Part model, mm, in its own coordinate system. Face numbers are marked on the shaded views. A direction names the side the tool comes from. Give positions to 0.01 mm unless a question says otherwise; leave off trailing zeros. Write each loop counter-clockwise with the first axis right and the second up, starting at its lowest first coordinate (ties: lowest second). Pieces come first, ordered by that corner, then holes. Notation, with made-up numbers: (60.5, 75.25) - (107.5, 75.25) arc R32 cw to (107.5, 108.25) - close; hole circle Ø5 at (74.5, 43). An arc over 180 degrees is marked (long way). Answer in a Markdown table with one row per item. Add a question column.
1. Drop flat-ended pins along their axis: pin 1 Ø4.5 at (x, y) = (0, 0) entering from +Z; pin 2 Ø5 at (x, y) = (0, 0) entering from -Z; pin 3 Ø3 at (y, z) = (12.5, -0.5) entering from -X. Give the stop position or say it passes through.
2. Band-saw the part on A-A on z = -2. Write the cut outline in (x, y).
3. Probe line 1 along Y through (x, z) = (0, 4.05); line 2 along Y through (x, z) = (0, 5.6); line 3 along X through (y, z) = (0, 3.25). List the from-to ranges inside material, lowest first.
4. Which spindle directions (+Z, -Z, +X, -X, +Y, -Y) get a long thin tool onto all of the face, cutting with end or side? Do the marked faces 1 and 2. Say none if no direction does.
5. Band-saw the part on C-C on x = -14.5. Write the cut outline in (y, z).
6. Pull direction Y, two halves, no side cores. Call the marked faces 3, 4 and 5: released by +Y, released by -Y, zero draft, split by the parting line, or undercut.
7. Band-saw the part on B-B on z = 5.5. Write the cut outline in (x, y), plus the area to 3 significant figures.
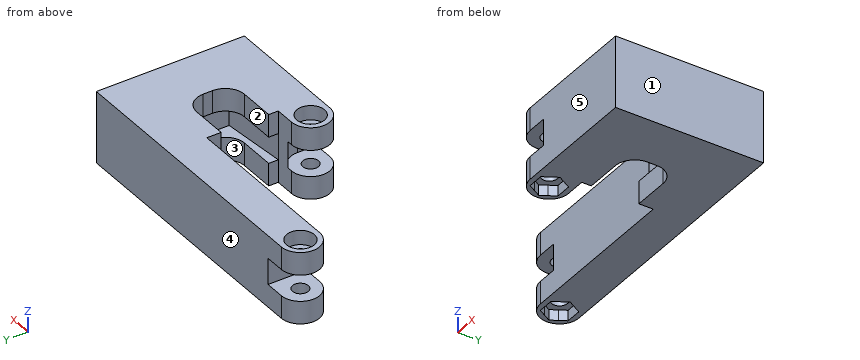
```python
from build123d import *

# Parameters (mm, degrees)
BOSS_EXTRUDE1_DEPTH      = 4.75
BOSS_EXTRUDE1_DEPTH_BACK = 4.75
SKETCH1_R                = 1.65
BOSS_EXTRUDE3_START      = -7.5
BOSS_EXTRUDE3_OUTLINE_R  = 1.65
BOSS_EXTRUDE3_DEPTH      = 15
CUT_EXTRUDE1_START       = -2.75
CUT_EXTRUDE1_OUTLINE_R   = 1.65
CUT_EXTRUDE1_DEPTH       = 5.5
CUT_EXTRUDE2_REACH       = 117.308
SKETCH3_W                = 5.5
SKETCH3_H                = 14
FILLET1_R                = 4
CUT_EXTRUDE3_START       = 7.5
SKETCH4_R                = 2.9
CUT_EXTRUDE3_DEPTH       = 3
CUT_EXTRUDE4_START       = -5.3
SKETCH4_4_R              = 2.9
CUT_EXTRUDE4_DEPTH       = 2.2


# Read off the part's stored shape, not the designer's step: Boss-Extrude3, Cut-Extrude1
with BuildPart() as part:
    # Sketch1 → Boss-Extrude1 (new, two sides: drawn at the far end of the back side and taken through both)
    with BuildSketch(Plane.XY.offset(-BOSS_EXTRUDE1_DEPTH_BACK)):
        with BuildLine():
            ThreePointArc((0, 4), (-4, 0), (0, -4))
            Line((0, -4), (26.73, -4))
            Line((26.73, -4), (26.73, 26.95))
            Line((26.73, 26.95), (-31.15, 26.95))
            ThreePointArc((-31.15, 26.95), (-35.15, 22.95), (-31.15, 18.95))
            Line((-31.15, 18.95), (4.15, 18.95))
            Line((4.15, 18.95), (4.15, 15.95))
            Line((4.15, 15.95), (15.73, 15.95))
            Line((15.73, 15.95), (15.73, 6))
            Line((15.73, 6), (4.15, 6))
            Line((4.15, 6), (4.15, 4))
            Line((4.15, 4), (0, 4))
        make_face()
        Circle(SKETCH1_R, mode=Mode.SUBTRACT)
        Polygon((-27.685898385, 22.95), (-29.417949192, 19.95), (-32.882050808, 19.95), (-34.614101615, 22.95), (-32.882050808, 25.95), (-29.417949192, 25.95), align=None, mode=Mode.SUBTRACT)
    extrude(amount=BOSS_EXTRUDE1_DEPTH + BOSS_EXTRUDE1_DEPTH_BACK)

    # Boss-Extrude3 outline → Boss-Extrude3 (add)
    with BuildSketch(Plane.XY.offset(BOSS_EXTRUDE3_START)):
        with BuildLine():
            Line((4.15, 4), (0, 4))
            ThreePointArc((0, 4), (-4, 0), (0, -4))
            Line((0, -4), (26.73, -4))
            Line((26.73, -4), (26.73, 26.95))
            Line((26.73, 26.95), (-31.15, 26.95))
            ThreePointArc((-31.15, 26.95), (-35.15, 22.95), (-31.15, 18.95))
            Line((-31.15, 18.95), (4.15, 18.95))
            Line((4.15, 18.95), (4.15, 15.95))
            Line((4.15, 15.95), (15.73, 15.95))
            Line((15.73, 15.95), (15.73, 6))
            Line((15.73, 6), (4.15, 6))
            Line((4.15, 6), (4.15, 4))
        make_face()
        Circle(BOSS_EXTRUDE3_OUTLINE_R, mode=Mode.SUBTRACT)
        with Locations((-31.15, 22.95)):
            Circle(BOSS_EXTRUDE3_OUTLINE_R, mode=Mode.SUBTRACT)
    extrude(amount=BOSS_EXTRUDE3_DEPTH)

    # Cut-Extrude1 outline → Cut-Extrude1 (cut)
    # profile 1 of 2: a face of its own
    with BuildSketch(Plane.XY.offset(CUT_EXTRUDE1_START)):
        with BuildLine():
            Line((0, -4), (4.15, -4))
            Line((4.15, -4), (4.15, 0))
            ThreePointArc((4.15, 0), (3.302349085, 2.513362393), (1.105667219, 4))
            Line((1.105667219, 4), (0, 4))
            ThreePointArc((0, 4), (-4, 0), (0, -4))
        make_face()
        Circle(CUT_EXTRUDE1_OUTLINE_R, mode=Mode.SUBTRACT)
    # profile 2 of 2: a face of its own
    with BuildSketch(Plane.XY.offset(CUT_EXTRUDE1_START)):
        with BuildLine():
            Line((-27, 18.95), (-27, 26.95))
            Line((-27, 26.95), (-31.15, 26.95))
            ThreePointArc((-31.15, 26.95), (-35.15, 22.95), (-31.15, 18.95))
            Line((-31.15, 18.95), (-27, 18.95))
        make_face()
        with Locations((-31.15, 22.95)):
            Circle(CUT_EXTRUDE1_OUTLINE_R, mode=Mode.SUBTRACT)
    extrude(amount=CUT_EXTRUDE1_DEPTH, mode=Mode.SUBTRACT)

    # Cut-Extrude2: up to this plane
    cut_extrude2_end = Plane(origin=(17.73, 0, -4.75), z_dir=(-1, 0, 0))
    # Sketch3 → Cut-Extrude2 (cut, up to the surface)
    with BuildSketch(Plane(origin=(-4.830790631, 106.650906635, 0), x_dir=(0, 0, -1), z_dir=(-0.9961946980917455, -0.08715574274765839, 0)), mode=Mode.PRIVATE) as cut_extrude2_sk1:
        with Locations((0, 96.043016422)):
            Rectangle(SKETCH3_W, SKETCH3_H)
    cut_extrude2_tool1 = split(extrude(cut_extrude2_sk1.sketch, amount=-CUT_EXTRUDE2_REACH, mode=Mode.PRIVATE), bisect_by=cut_extrude2_end, keep=Keep.BOTH, mode=Mode.PRIVATE)
    add(cut_extrude2_tool1.solids().sort_by_distance((3.53991, 10.973363, 0))[0], mode=Mode.SUBTRACT)

    # Fillet1
    fillet1_edges = [part.edges().sort_by_distance(p)[0] for p in [
        (15.73, 6, 5.125),
        (15.73, 15.95, 5.125),
        (15.73, 6, -5.125),
        (15.73, 15.95, -5.125),
    ]]
    fillet(fillet1_edges, radius=FILLET1_R)

    # Sketch4 → Cut-Extrude3 (cut)
    with BuildSketch(Plane.XY.offset(CUT_EXTRUDE3_START)):
        with Locations((-31.15, 22.95)):
            Circle(SKETCH4_R)
        Circle(SKETCH4_R)
    extrude(amount=-CUT_EXTRUDE3_DEPTH, mode=Mode.SUBTRACT)

    # Sketch4<4> → Cut-Extrude4 (cut)
    with BuildSketch(Plane.XY.offset(CUT_EXTRUDE4_START)):
        Circle(SKETCH4_4_R)
        with BuildLine():
            Line((-1.674315781, -2.9), (0, -2.9))
            ThreePointArc((0, -2.9), (-1.450000053, -2.511473641), (-2.511473732, -1.449999895))
            Line((-2.511473732, -1.449999895), (-1.674315781, -2.9))
        make_face()
        with BuildLine():
            ThreePointArc((-2.511473732, -1.449999895), (-2.9, 9e-09), (-2.511473723, 1.44999991))
            Line((-2.511473723, 1.44999991), (-3.348631561, 0))
            Line((-3.348631561, 0), (-2.511473732, -1.449999895))
        make_face()
        with BuildLine():
            ThreePointArc((-2.511473723, 1.44999991), (-1.45000005, 2.511473642), (-1.2e-08, 2.9))
            Line((-1.2e-08, 2.9), (-1.674315781, 2.9))
            Line((-1.674315781, 2.9), (-2.511473723, 1.44999991))
        make_face()
        with BuildLine():
            ThreePointArc((-1.2e-08, 2.9), (1.449999995, 2.511473674), (2.511473671, 1.45))
            Line((2.511473671, 1.45), (1.674315781, 2.9))
            Line((1.674315781, 2.9), (-1.2e-08, 2.9))
        make_face()
        with BuildLine():
            Line((2.511473679, -1.449999986), (3.348631561, 0))
            Line((3.348631561, 0), (2.511473671, 1.45))
            ThreePointArc((2.511473671, 1.45), (2.801184896, 0.750575231), (2.9, 0))
            ThreePointArc((2.9, 0), (2.801184898, -0.750575223), (2.511473679, -1.449999986))
        make_face()
        with BuildLine():
            Line((1.674315781, -2.9), (2.511473679, -1.449999986))
            ThreePointArc((2.511473679, -1.449999986), (1.450000007, -2.511473667), (0, -2.9))
            Line((0, -2.9), (1.674315781, -2.9))
        make_face()
        with Locations((-31.15, 22.95)):
            Circle(SKETCH4_4_R)
        with BuildLine():
            Line((-29.475684219, 20.05), (-28.638526291, 21.500000065))
            ThreePointArc((-28.638526291, 21.500000065), (-29.699999968, 20.438526348), (-31.15, 20.05))
            Line((-31.15, 20.05), (-29.475684219, 20.05))
        make_face()
        with BuildLine():
            Line((-28.638526291, 21.500000065), (-27.801368439, 22.95))
            Line((-27.801368439, 22.95), (-28.638526352, 24.40000004))
            ThreePointArc((-28.638526352, 24.40000004), (-28.34881511, 23.700575253), (-28.25, 22.95))
            ThreePointArc((-28.25, 22.95), (-28.348815094, 22.199424805), (-28.638526291, 21.500000065))
        make_face()
        with BuildLine():
            ThreePointArc((-31.150000038, 25.85), (-29.700000036, 25.461473692), (-28.638526352, 24.40000004))
            Line((-28.638526352, 24.40000004), (-29.475684219, 25.85))
            Line((-29.475684219, 25.85), (-31.150000038, 25.85))
        make_face()
        with BuildLine():
            ThreePointArc((-33.661473709, 24.399999935), (-32.600000049, 25.461473643), (-31.150000038, 25.85))
            Line((-31.150000038, 25.85), (-32.824315781, 25.85))
            Line((-32.824315781, 25.85), (-33.661473709, 24.399999935))
        make_face()
        with BuildLine():
            ThreePointArc((-33.661473549, 21.499999789), (-34.05, 22.949999841), (-33.661473709, 24.399999935))
            Line((-33.661473709, 24.399999935), (-34.498631561, 22.95))
            Line((-34.498631561, 22.95), (-33.661473549, 21.499999789))
        make_face()
        with BuildLine():
            Line((-32.824315781, 20.05), (-31.15, 20.05))
            ThreePointArc((-31.15, 20.05), (-32.599999895, 20.438526268), (-33.661473549, 21.499999789))
            Line((-33.661473549, 21.499999789), (-32.824315781, 20.05))
        make_face()
    extrude(amount=-CUT_EXTRUDE4_DEPTH, mode=Mode.SUBTRACT)


solid = part.part
```
Values:
| question | item | result |
|---|---|---|
| 1 | pin 1 | stops at z = 4.5 |
| 1 | pin 2 | stops at z = -5.3 |
| 1 | pin 3 | stops at x = 17.73 |
| 2 | outline | (-27, 18.95) - (4.15, 18.95) - (4.15, 18.05) - (17.73, 19.24) - (17.73, 5.19) - (4.15, 4) - (1.11, 4) arc R4.15 cw to (4.15, 0) - (4.15, -4) - (26.73, -4) - (26.73, 26.95) - (-27, 26.95) - close |
| 3 | line 1 | y = -4 to -1.65, 1.65 to 4, 18.95 to 26.95 |
| 3 | line 2 | y = -4 to -2.9, 2.9 to 4, 18.95 to 26.95 |
| 3 | line 3 | x = -4 to -1.65, 1.65 to 26.73 |
| 4 | face 1 | +Z, -Z, +X, +Y, -Y |
| 4 | face 2 | +Z, -Z, -X |
| 5 | outline | (18.95, -7.5) - (26.95, -7.5) - (26.95, 7.5) - (18.95, 7.5) - close |
| 6 | face 3 | undercut |
| 6 | face 4 | released by +Y |
| 6 | face 5 | released by -Y |
| 7 | outline | (-31.15, 18.95) - (4.15, 18.95) - (4.15, 15.95) - (11.73, 15.95) arc R4 cw to (15.73, 11.95) - (15.73, 10) arc R4 cw to (11.73, 6) - (4.15, 6) - (4.15, 4) - (0, 4) arc R4 ccw to (0, -4) - (26.73, -4) - (26.73, 26.95) - (-31.15, 26.95) arc R4 ccw to start; hole circle Ø5.8 at (-31.15, 22.95); hole circle Ø5.8 at (0, 0) |
| 7 | area | 904 mm² |
